Verification items for this drawing (mm, ordinates from the low corner). A direction names the side the tool comes from. Coordinates: 2 decimals unless noted, no trailing zeros. Loops run counter-clockwise (first coordinate to the right, second up) from the corner with the lowest first, then second, coordinate; pieces in that order, holes last. Notation, with made-up numbers: (57.25, 46.25) - (66.25, 46.25) arc R35 cw to (66.25, 79.25) - close; hole circle Ø10 at (5, 36). An arc over 180 degrees is marked (long way). One line per item, written item: value. Start each with the question number.
(1) Section check D-D (x = 16.5). Record the boundary of the cut face in (y, z).
(2) Section check A-A (x = 7.5). Record the boundary of the cut face in (y, z), plus the area to 3 significant figures.
(3) Draft check along Z on the marked faces 1, 2, 3 and 4. Enter one of: +Z half, -Z half, draft (parallel to the pull), parting line (faces both ways), or undercut.
(4) Thickness scan on probe 1 along X at (y, z) = (26.8, 3); probe 2 along Z at (x, y) = (17, 28.3); probe 3 along Z at (x, y) = (6.5, 11.5). Record the ranges inside material, lowest first. Write a range as [from, to].
(5) Set-up check for the marked faces 5, 6 and 7: record each of +Z, -Z, +X, -X, +Y, -Y from which the full face is reachable in a straight line by a thin tool's end or side.
(6) Section check B-B (z = 4.5). Record the boundary of the cut face in (x, y), plus the area to 3 significant figures.
(7) Section check C-C (y = 22). Record the boundary of the cut face in (x, z).
(8) Gauge pin test, flat ends, axial feed: P1, Ø2, axis at y = 28.5, z = 8.5, coming from the -X side; P2, Ø4.5, axis at x = 11.5, y = 15.5, coming from the +Z side; P3, Ø5, axis at y = 18, z = 3.5, coming from the +X side; P4, Ø3.5, axis at x = 3, z = 3, coming from the -Y side. Record the tip position at first contact, or that the pin passes through.
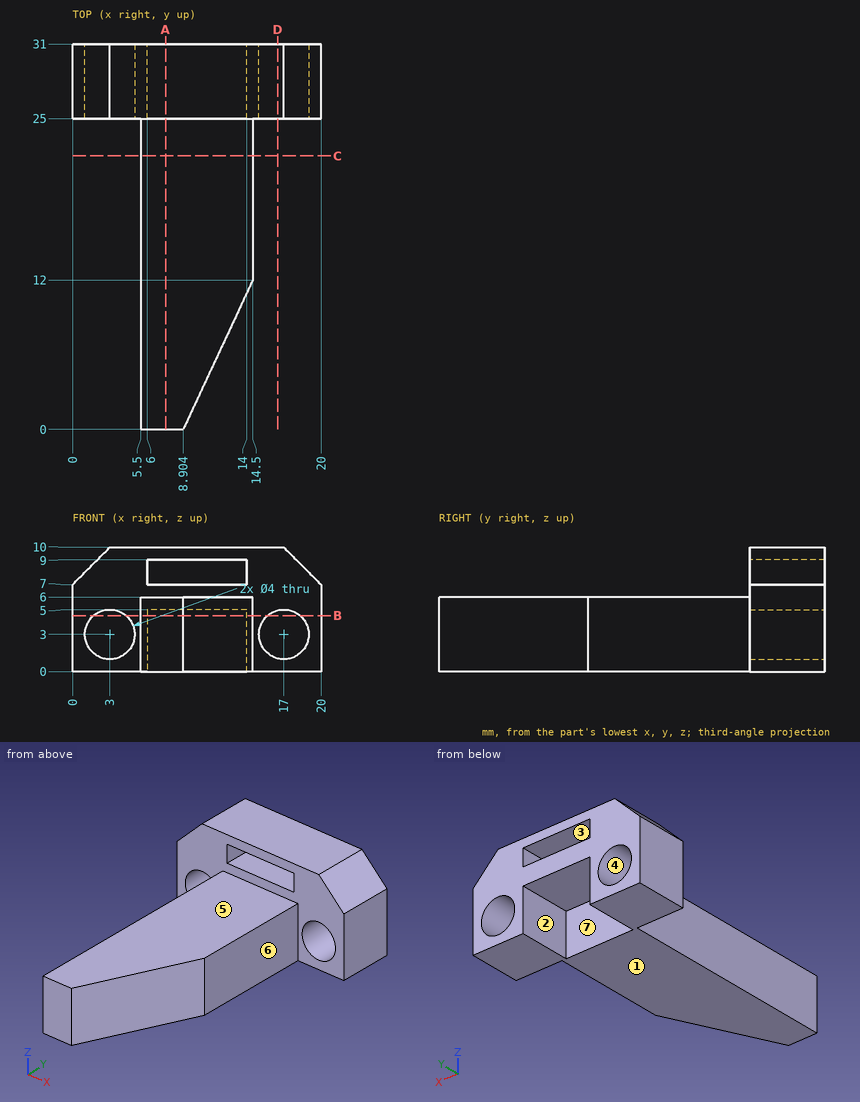
Responses:
1. outline: (25, 0) - (31, 0) - (31, 1.06) - (25, 1.06) - close; (25, 4.94) - (31, 4.94) - (31, 10) - (25, 10) - close
2. outline: (0, 0) - (25, 0) - (25, 5) - (31, 5) - (31, 7) - (25, 7) - (25, 6) - (0, 6) - close; (25, 9) - (31, 9) - (31, 10) - (25, 10) - close
2. area: 168 mm²
3. face 1: -Z half
3. face 2: draft
3. face 3: undercut
3. face 4: undercut
4. probe 1: x = [0, 1], [5, 6], [14, 15], [19, 20]
4. probe 2: z = [0, 1], [5, 10]
4. probe 3: z = [0, 6]
5. face 5: +Z, +X, -X, -Y
5. face 6: +Z, -Z, +X, -Y
5. face 7: -Z, +Y
6. outline: (0, 25) - (1.68, 25) - (1.68, 31) - (0, 31) - close; (4.32, 25) - (5.5, 25) - (5.5, 0) - (8.9, 0) - (14.5, 12) - (14.5, 25) - (15.68, 25) - (15.68, 31) - (14, 31) - (14, 25) - (6, 25) - (6, 31) - (4.32, 31) - close; (18.32, 25) - (20, 25) - (20, 31) - (18.32, 31) - close
6. area: 232 mm²
7. outline: (5.5, 0) - (14.5, 0) - (14.5, 6) - (5.5, 6) - close
8. P1: stops at x = 0.5
8. P2: stops at z = 6
8. P3: stops at x = 14.5
8. P4: passes through
